Design review of the part built by this model. Coordinates are the model's own, in mm. A direction names the side the tool comes from. Give positions to 0.01 mm unless a question says otherwise; leave off trailing zeros. Loops run counter-clockwise (first coordinate to the right, second up) from the corner with the lowest first, then second, coordinate; pieces in that order, holes last. Notation, with made-up numbers: (65.5, 24) - (79.5, 24) arc R21 cw to (79.5, 49) - close; hole circle Ø4 at (69, 75). An arc over 180 degrees is marked (long way). Write each question's results on one line, items separated by ' | '.
Autodesk Inventor part; units mm, degrees
ref_plane "YZ Plane" through (0, 0, 0) normal (1, 0, 0) x (0, 1, 0)
ref_plane "XZ Plane" through (0, 0, 0) normal (0, 1, 0) x (-1, 0, 0)
ref_plane "XY Plane" through (0, 0, 0) normal (0, 0, 1) x (1, 0, 0)
sketch "Sketch1" plane through (0, 0, 0) normal (0, 0, 1) x (1, 0, 0)
  line L0 (0, -9.797) -> (50, -9.797)
  line L1 (0, -9.797) -> (-50, -9.797)
  line L2 (50, -9.797) -> (30, -9.797)
  line L3 (30, 30.203) -> (50, -9.797)
  line L4 (-50, 30.203) -> (30, 30.203)
  line L5 (-50, -9.797) -> (-54, -9.797)
  line L6 (-50, 30.203) -> (-54, 30.203)
  line L7 (-54, -9.797) -> (-54, 30.203)
  point P0 (0, 0)
  dimension "d4" = 20
  dimension "d5" = 40
  dimension "d27" = 104
  dimension "d29" = 84
extrude "Extrusion3" add sketch "Sketch1" along normal blind 5
sketch "Sketch3" plane through (-54, -9.797, 0) normal (0, -1, 0) x (1, 0, 0)
  line L0 (104, 0) -> (104, 5) construction
  line L1 (104, 5) -> (81.5, 5) construction
  line L2 (84, 5) -> (0, 5) construction
  line L3 (81.5, 5) -> (66.5, 5)
  line L4 (66.5, 5) -> (66.5, 2)
  line L5 (66.5, 2) -> (81.5, 2)
  line L6 (81.5, 2) -> (81.5, 5)
  line L7 (66.5, 5) -> (66.5, 3) construction
  line L8 (31.5, 2) -> (16.5, 2)
  line L9 (16.5, 2) -> (16.5, 5)
  line L10 (16.5, 5) -> (31.5, 5)
  line L11 (31.5, 5) -> (31.5, 2)
  circle A0 centre (49, 3) radius 1.75
  point P0 (54, 0)
  dimension "d32" = 22.5
  dimension "d33" = 15
  dimension "d34" = 3
  dimension "d41" = 15
  dimension "d42" = 3
  dimension "d44" = 3.5
  dimension "d45" = 15.75
  dimension "d46" = 17.5
extrude "Extrusion4" add sketch "Sketch3" along normal blind 3 contours L6 L5 L4 L3 | L8 L9 L10 L11
extrude "Extrusion5" cut sketch "Sketch3" against normal blind 15 contours A0
equation "\"d41\" = d33"
equation "\"d42\" = d34"
properties part number "latera_trapezio_agitador"
(1) Take a section at D-D on x = 15. Give the boundary of the cut face in (y, z).
Answers below:
outline: (-12.8, 2) - (-9.8, 2) - (-9.8, 0) - (30.2, 0) - (30.2, 5) - (-12.8, 5) - close
(2) Insertion check: P1, Ø2.5, axis at y = -11, z = 3, coming from the -X side; P2, Ø0.9, axis at y = -11.5, z = 3, coming from the -X side; P3, Ø1.8, axis at x = -5, z = 3, coming from the -Y side; P4, Ø2.5, axis at y = -11.5, z = 4, coming from the +X side. Each pin has a flat end and moves straight along its axis. Give the tip position at first contact, or say it passes through.
Answers below:
P1: x = -54 | P2: x = -37.5 | P3: y = 5.2 | P4: x = 27.5
(3) Take a section at A-A on x = -5. Give the boundary of the cut face in (y, z).
Answers below:
outline: (-9.8, 0) - (30.2, 0) - (30.2, 5) - (-9.8, 5) - (-9.8, 4.75) - (5.2, 4.75) - (5.2, 1.25) - (-9.8, 1.25) - close
(4) Take a section at C-C on z = 3. Give the boundary of the cut face in (x, y).
Answers below:
outline: (-54, -9.8) - (-37.5, -9.8) - (-37.5, -12.8) - (-22.5, -12.8) - (-22.5, -9.8) - (-6.75, -9.8) - (-6.75, 5.2) - (-3.25, 5.2) - (-3.25, -9.8) - (12.5, -9.8) - (12.5, -12.8) - (27.5, -12.8) - (27.5, -9.8) - (50, -9.8) - (30, 30.2) - (-54, 30.2) - close
(5) Take a section at B-B on y = -3. Give the boundary of the cut face in (x, z).
Answers below:
outline: (-54, 0) - (46.6, 0) - (46.6, 5) - (-54, 5) - close; hole circle Ø3.5 at (-5, 3)
(6) Wall thickness on line 1 along Z through (x, y) = (-5, -2); line 2 along Y through (x, z) = (-27.5, 0.35); line 3 along Z through (x, y) = (-23.5, -10): over which ranges is each line inside the solid? List them lowest first. Write a range as from..to.
Answers below:
line 1: 0..1.25, 4.75..5 | line 2: -9.8..30.2 | line 3: 2..5
(7) Tool access review of faces 4 (the flat face through (-3, 10, 0)), 5 (the flat face through (27.5, -11, 3)), 6 (the flat face through (12.5, -11, 4)), 7 (the flat face through (20, -11, 2)), 8 (the flat face through (-5, 5.203, 3)): name each direction out of +Z, -Z, +X, -X, +Y, -Y from which nothing blocks a thin tool from reaching the whole face with its end or side.
Answers below:
face 4: -Z, +X, -X, +Y, -Y | face 5: +Z, -Z, +X, -Y | face 6: +Z, -Z, -Y | face 7: -Z, +X, -X, -Y | face 8: -Y
(8) Draft analysis for pull direction X (two halves, no side actions). For faces 1 (the flat face through (-30, -11, 2)), 2 (the flat face through (-37.5, -11, 3)), 3 (the flat face through (-22.5, -11, 4)), state which applies: pulls with the +X half, pulls with the -X half, needs draft (parallel to the pull), parting line crosses it, or undercut.
Answers below:
face 1: needs draft | face 2: pulls with the -X half | face 3: undercut
